Autodesk Inventor part; units mm, degrees
ref_plane "YZ Plane" through (0, 0, 0) normal (1, 0, 0) x (0, 1, 0)
ref_plane "XZ Plane" through (0, 0, 0) normal (0, 1, 0) x (-1, 0, 0)
ref_plane "XY Plane" through (0, 0, 0) normal (0, 0, 1) x (1, 0, 0)
sketch "Sketch1" plane through (0, 0, 0) normal (1, 0, 0) x (0, 1, 0)
  line L0 (0, 0) -> (-475.5283, 154.5085)
  line L1 (0, 0) -> (500, 0) construction
  line L2 (-470.584, 169.7254) -> (2.5342, 16)
  line L3 (2.5342, 16) -> (500, 16)
  line L4 (0, 0) -> (0, 16.8234)
  line L5 (-470.584, 169.7254) -> (-470.584, 152.902)
  dimension "d0" = 500
  dimension "d1" = 162
  dimension "d2" = 16
extrude "Extrusion1" add sketch "Sketch1" along normal blind 16
fillet "Fillet1" radius 8 4 edges at (16, -235.292, 76.451) (0, -235.292, 76.451) (16, -235.292, 93.2744) (0, -235.292, 93.2744)
properties part number "Leg_Mockup"
Can you work these out from the model? Positions are in its coordinate system, mm. Round coordinates to 2 decimals unless told otherwise and drop trailing zeros. Loops run counter-clockwise (first coordinate to the right, second up) from the corner with the lowest first, then second, coordinate; pieces in that order, holes last. Notation, with made-up numbers: (55.5, 55.5) -> (81.5, 55.5) arc R15 ccw to (81.5, 82.5) -> close; hole circle Ø8 at (45, 43). An arc over 180 degrees is marked (long way). Answer in a Markdown table with one row per item.
Item 1: Will these pins go through, and if not, where does the flat tip stop? P1, Ø8, axis at x = 3.5, y = -70, coming from the +Z side; P2, Ø4, axis at x = 5, y = -273.5, coming from the +Z side; P3, Ø5, axis at x = 2.5, y = -233.5, coming from the -Z side.
Answer block:
| item | result |
|---|---|
| P1 | z = 40.32 |
| P2 | z = 105.99 |
| P3 | z = 76.23 |
Item 2: Suppose I cut it at A-A, the plane x = 10.75. List the corners of the cut face in (y, z) for me.
Answer block:
| item | result |
|---|---|
| outline | (-470.58, 153.41) -> (0, 0.51) -> (0, 16.31) -> (-470.58, 169.21) -> close |
Item 3: If I drill on probe 1 along Z at (x, y) = (9.5, -54); probe 2 along Z at (x, y) = (2.25, -385.5); probe 3 along X at (y, z) = (-340.5, 115), over which ranges is the centre line in solid material (lowest first)?
Answer block:
| item | result |
|---|---|
| probe 1 | 17.69 to 34.22 |
| probe 2 | 127.82 to 139.52 |
| probe 3 | 0.99 to 15.01 |
